from build123d import *

# Parameters (mm, degrees)
SKETCH2_W               = 12.7
SKETCH2_H               = 12.7
SKETCH1_W               = 15.748
SKETCH1_H               = 15.748
CUT_EXTRUDE1_DEPTH      = 8.8740001
CUT_EXTRUDE1_DEPTH_BACK = 8.8740001
FILLET1_R               = 0.254


with BuildPart() as part:
    # Sketch2 → Loft1 section 0
    with BuildSketch(Plane(origin=(0, 15.24, 0), x_dir=(1, 0, 0), z_dir=(0, 1, 0))):
        Rectangle(SKETCH2_W, SKETCH2_H)
    # Sketch1 → Loft1 section 1
    with BuildSketch(Plane(origin=(0, 0, 0), x_dir=(1, 0, 0), z_dir=(0, 1, 0))):
        Rectangle(SKETCH1_W, SKETCH1_H)
    loft()

    # Sketch3 → Cut-Extrude1 (cut, two sides)
    with BuildSketch(Plane.XY) as cut_extrude1_sk:
        with BuildLine():
            Line((-56.40168157, 28.163288611), (-6.35, 15.24))
            ThreePointArc((-6.35, 15.24), (0, 14.433444248), (6.35, 15.24))
            Line((6.35, 15.24), (56.40168157, 28.163288611))
            Line((56.40168157, 28.163288611), (56.40168157, 131.549597501))
            Line((56.40168157, 131.549597501), (-56.40168157, 131.549597501))
            Line((-56.40168157, 131.549597501), (-56.40168157, 28.163288611))
        make_face()
    extrude(amount=CUT_EXTRUDE1_DEPTH, mode=Mode.SUBTRACT)
    extrude(cut_extrude1_sk.sketch, amount=-CUT_EXTRUDE1_DEPTH_BACK, mode=Mode.SUBTRACT)

    # Fillet1
    fillet1_edges = [part.edges().sort_by_distance(p)[0] for p in [
        (6.35, 15.24, 0),
        (-6.35, 15.24, 0),
    ]]
    fillet(fillet1_edges, radius=FILLET1_R)


solid = part.part
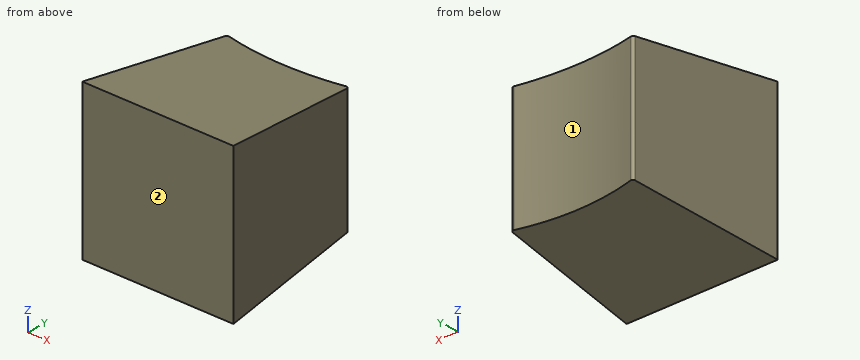
Design review of the part built by this model. Coordinates are the model's own, in mm. Face numbers are marked on the shaded views. Coordinates: 2 decimals unless noted, no trailing zeros. Use one line per item in the form item = value.
(1) For line 1 along Y through (x, z) = (0.25, -1.25); line 2 along Y through (x, z) = (6.25, 5.5); line 3 along X through (y, z) = (1, 2.5), list the stretches that pass through material, from the lowest coordinate up. Write a range as from..to.
Return value:
line_1 = 0..14.43
line_2 = 0..15.14
line_3 = -7.77..7.77
(2) Draft analysis for pull direction X (two halves, no side actions). For the marked faces 1 and 2, state which applies: pulls with the +X half, pulls with the -X half, needs draft (parallel to the pull), parting line crosses it, or undercut.
Return value:
face_1 = undercut
face_2 = needs draft
(3) Clearance check with flat-ended pins moving along their axes: P1, Ø3, axis at x = -1, z = -3, coming from the +Y side; P2, Ø1.5, axis at x = -5, y = 11, coming from the -Z side; P3, Ø4, axis at x = 3, z = -2, coming from the +Y side; P4, Ø3, axis at x = -1, z = -4.5, coming from the -Y side. State where each tip first meets the part, or that it passes through.
Return value:
P1 = 14.56
P2 = -6.85
P3 = 14.93
P4 = 0
